from build123d import *

# Parameters (mm, degrees)
F1_DEPTH = 76.2
F3_DEPTH = 25.4
F5_DEPTH = 45.466
F6_R     = 38.1
F7_R     = 38.1


with BuildPart() as f1:
    # F0 (on Right) → F1 (new body, symmetric)
    with BuildSketch(Plane.YZ):
        Polygon((-76.2, 0), (0, 0), (0, 152.4), (-25.4, 152.4), (-25.4, 25.4), (-76.2, 25.4), align=None)
    extrude(amount=F1_DEPTH, both=True)

    # F2 (on face) → F3 (cut)
    with BuildSketch(Plane(origin=(0, 0, 0), x_dir=(-1, 0, 0), z_dir=(0, 1, 0))):
        with BuildLine():
            ThreePointArc((0, 127), (-8.980256, 105.319744), (12.7, 114.3))
            ThreePointArc((12.7, 114.3), (8.980256, 123.280256), (0, 127))
        make_face()
    extrude(amount=-F3_DEPTH, mode=Mode.SUBTRACT)

    # F4 (on face) → F5 (cut)
    with BuildSketch(Plane.XY.offset(25.4)):
        with BuildLine():
            Line((12.7, -76.2), (12.7, -63.5))
            ThreePointArc((12.7, -63.5), (0, -50.8), (-12.7, -63.5))
            Line((-12.7, -63.5), (-12.7, -76.2))
            Line((-12.7, -76.2), (12.7, -76.2))
        make_face()
    extrude(amount=-F5_DEPTH, mode=Mode.SUBTRACT)

    # F6
    f6_edges = [f1.edges().sort_by_distance(p)[0] for p in [
        (76.2, -12.7, 152.4),
    ]]
    fillet(f6_edges, radius=F6_R)

    # F7
    f7_edges = [f1.edges().sort_by_distance(p)[0] for p in [
        (-76.2, -12.7, 152.4),
    ]]
    fillet(f7_edges, radius=F7_R)


solid = f1.part
Can you work these out from the model? Positions are in its coordinate system, mm. A direction names the side the tool comes from. Round coordinates to 2 decimals unless told otherwise and drop trailing zeros. Order: outer loops, then holes, each group sorted by start corner. A loop starts at its lowest first (then second) coordinate and runs counter-clockwise, first axis right, second up. Notation, with made-up numbers: (37, 44) - (54, 44) arc R17 ccw to (54, 57) - close; hole circle Ø8 at (-10.75, 68). An arc over 180 degrees is marked (long way). Answer in a Markdown table with one row per item.
(1) Suppose I cut it at B-B, the plane y = -57. Please give me the cut outline in (x, z).
From the geometry:
| item | result |
|---|---|
| outline | (-76.2, 0) - (-10.91, 0) - (-10.91, 25.4) - (-76.2, 25.4) - close; (10.91, 0) - (76.2, 0) - (76.2, 25.4) - (10.91, 25.4) - close |
(2) Please list where these lines run through material, in increasing order: L1, parallel to Z at x = 1, y = -7; L2, parallel to Y at x = -31.5, z = 47; L3, parallel to X at y = -5, z = 114. Write a range as from..to.
From the geometry:
| item | result |
|---|---|
| L1 | z = 0..101.64, 126.96..152.4 |
| L2 | y = -25.4..0 |
| L3 | x = -76.2..-12.7, 12.7..76.2 |
(3) Suppose I cut it at C-C, the plane z = 43. Please give me the cut outline in (x, y).
From the geometry:
| item | result |
|---|---|
| outline | (-76.2, -25.4) - (76.2, -25.4) - (76.2, 0) - (-76.2, 0) - close |
(4) Which directions (+Z, -Z, +X, -X, +Y, -Y) give clear straight access to the entire face, cutting with the end or side of a thin tool? Please do faces 1 (the face through (1, -50, 25.4)), 2 (the face through (-44, -76.2, 13)), 3 (the face through (12.7, -70, 13)).
From the geometry:
| item | result |
|---|---|
| face 1 | +Z, +X, -X, -Y |
| face 2 | +Z, -Z, +X, -X, -Y |
| face 3 | +Z, -Z, -Y |
(5) For P1, Ø1, axis at x = 51.5, z = 54, coming from the -Y side; P2, Ø15, axis at x = 4, y = -53.5, coming from the +Z side; P3, Ø1.5, axis at x = -41, y = -23, coming from the -Z side; P4, Ø5, axis at x = 61, y = -18, coming from the +Z side, each with a flat end and sliding along its axis, tell me the tip position at first contact or that it passes through.
From the geometry:
| item | result |
|---|---|
| P1 | stops at y = -25.4 |
| P2 | stops at z = 25.4 |
| P3 | stops at z = 0 |
| P4 | stops at z = 146.48 |
(6) Suppose I cut it at D-D, the plane y = -38. Please give me the cut outline in (x, z), plus the area to 3 significant figures.
From the geometry:
| item | result |
|---|---|
| outline | (-76.2, 0) - (76.2, 0) - (76.2, 25.4) - (-76.2, 25.4) - close |
| area | 3,870 mm2 |
(7) Suppose I cut it at A-A, the plane x = -23.5. Please give me the cut outline in (y, z), plus the area to 3 significant figures.
From the geometry:
| item | result |
|---|---|
| outline | (-76.2, 0) - (0, 0) - (0, 152.4) - (-25.4, 152.4) - (-25.4, 25.4) - (-76.2, 25.4) - close |
| area | 5,160 mm2 |
(8) If we mould it in two halves opening along X, with no side actions, what happens to faces 4 (the face through (-12.7, -70, 13)), 5 (the face through (65.34, -12.88, 140.94)), 6 (the face through (-76.2, -22, 45))? For each: released by +X, released by -X, zero draft, split by the parting line, or undercut.
From the geometry:
| item | result |
|---|---|
| face 4 | undercut |
| face 5 | released by +X |
| face 6 | released by -X |
